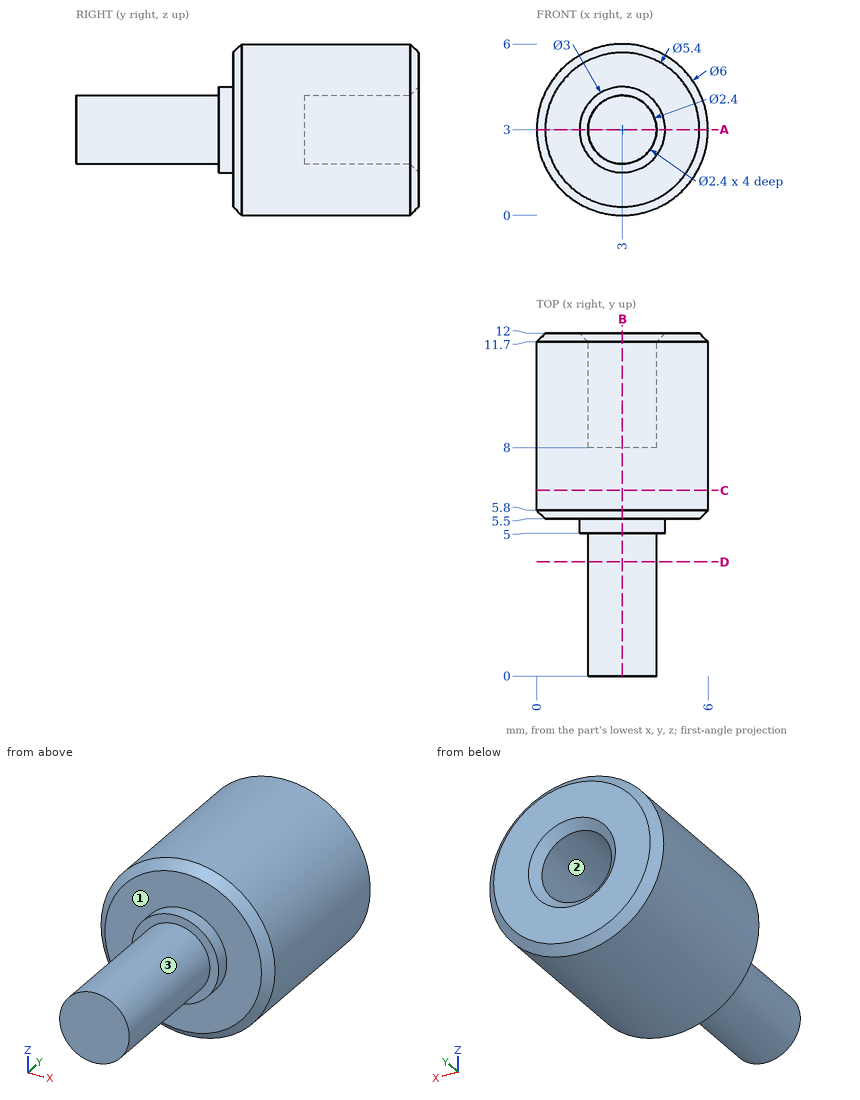
Geometry: see drawing. Coordinates: mm, zero at the bounding-box minimum. Coordinates: 2 decimals unless noted, no trailing zeros. Loops run counter-clockwise (first coordinate to the right, second up) from the corner with the lowest first, then second, coordinate; pieces in that order, holes last. Notation, with made-up numbers: (61.5, 59.25) - (108.5, 59.25) arc R17 cw to (108.5, 84.25) - close; hole circle Ø2 at (0, 63). An arc over 180 degrees is marked (long way). Answer in a Markdown table with one row per item.
(1) Pin query (flat end, axial travel): P1, Ø1, axis at x = 5, y = 8, coming from the -Z side; P2, Ø1.9, axis at x = 3, z = 3, coming from the +Y side. Return the tip coordinate at first contact, or that it passes through.
Model answer:
| item | result |
|---|---|
| P1 | stops at z = 0.4 |
| P2 | stops at y = 8 |
(2) Cut plane C-C on y = 6.5. Output: boundary loops of the cut face in (x, z).
Model answer:
| item | result |
|---|---|
| outline | circle Ø6 at (3, 3) |
(3) Material intervals for L1, parallel to Z at x = 3, y = 9.1; L2, parallel to Y at x = 4.35, z = 1; L3, parallel to Y at x = 4.1, z = 3, sorted ascending. Write a range as from..to.
Model answer:
| item | result |
|---|---|
| L1 | z = 0..1.8, 4.2..6 |
| L2 | y = 5.5..12 |
| L3 | y = 0..8 |
(4) Cut plane A-A on z = 3. Output: boundary loops of the cut face in (x, y).
Model answer:
| item | result |
|---|---|
| outline | (0, 5.8) - (0.3, 5.5) - (1.5, 5.5) - (1.5, 5) - (1.8, 5) - (1.8, 0) - (4.2, 0) - (4.2, 5) - (4.5, 5) - (4.5, 5.5) - (5.7, 5.5) - (6, 5.8) - (6, 11.7) - (5.7, 12) - (4.5, 12) - (4.2, 11.7) - (4.2, 8) - (1.8, 8) - (1.8, 11.7) - (1.5, 12) - (0.3, 12) - (0, 11.7) - close |
(5) Cut plane D-D on y = 4. Output: boundary loops of the cut face in (x, z), plus the area to 3 significant figures.
Model answer:
| item | result |
|---|---|
| outline | circle Ø2.4 at (3, 3) |
| area | 4.52 mm² |
(6) Mould query, pull axis Z, two halves, no side actions, for the marked faces 1, 2 and 3. Classes: pulls with the +Z half, pulls with the -Z half, needs draft (parallel to the pull), parting line crosses it, or undercut.
Model answer:
| item | result |
|---|---|
| face 1 | needs draft |
| face 2 | undercut |
| face 3 | parting line crosses it |
(7) Cut plane B-B on x = 3. Output: boundary loops of the cut face in (y, z).
Model answer:
| item | result |
|---|---|
| outline | (0, 1.8) - (5, 1.8) - (5, 1.5) - (5.5, 1.5) - (5.5, 0.3) - (5.8, 0) - (11.7, 0) - (12, 0.3) - (12, 1.5) - (11.7, 1.8) - (8, 1.8) - (8, 4.2) - (11.7, 4.2) - (12, 4.5) - (12, 5.7) - (11.7, 6) - (5.8, 6) - (5.5, 5.7) - (5.5, 4.5) - (5, 4.5) - (5, 4.2) - (0, 4.2) - close |
